from build123d import *

# Parameters (mm, degrees)
BOSS_EXTRUDE1_DEPTH = 4.7498
SKETCH2_R           = 5.715
BOSS_EXTRUDE2_DEPTH = 4.7498
SKETCH3_W           = 112.522
SKETCH3_H           = 50.8
SKETCH3_W_2         = 88.835533053
BOSS_EXTRUDE3_DEPTH = 228.6


with BuildPart() as part:
    # Sketch1 → Boss-Extrude1 (new body)
    with BuildSketch(Plane(origin=(0, 0, 0), x_dir=(1, 0, 0), z_dir=(0, 1, 0))):
        Polygon((23.686466947, -292.1), (112.522, -292.1), (112.522, -139.7), (-61.722, 292.1), (-112.522, 292.1), (-112.522, 0), align=None)
    extrude(amount=BOSS_EXTRUDE1_DEPTH)



with BuildPart() as body_2:
    # Sketch2 → Boss-Extrude2 (new body)
    with BuildSketch(Plane(origin=(-112.522, 0, 11.737401462), x_dir=(0, 0, -1), z_dir=(1, 0, 0))):
        Polygon((176.837401462, 4.7498), (231.249840519, 42.8498), (303.837401462, 42.8498), (303.837401462, 4.7498), align=None)
        with Locations(Location((291.137401462, 23.7998, 0), (0, 0, 180))):
            Circle(SKETCH2_R, mode=Mode.SUBTRACT)
        with Locations(Location((240.337401462, 23.7998, 0), (0, 0, 180))):
            Circle(SKETCH2_R, mode=Mode.SUBTRACT)
    extrude(amount=BOSS_EXTRUDE2_DEPTH)


with BuildPart() as part_1:
    add(part.part)

    add(body_2.part)  # Boss-Extrude3 merges body 2
    # Sketch3 → Boss-Extrude3 (add)
    with BuildSketch(Plane(origin=(0, 4.7498, 0), x_dir=(1, 0, 0), z_dir=(0, 1, 0))):
        with Locations((-56.261, 139.7)):
            Rectangle(SKETCH3_W, SKETCH3_H)
        with Locations((68.104233474, -266.7)):
            Rectangle(SKETCH3_W_2, SKETCH3_H)
    extrude(amount=BOSS_EXTRUDE3_DEPTH)

    # Mirror1: part across plane


with BuildPart() as part_2:
    add(part_1.part)
    add(part_1.part.mirror(Plane.ZX.offset(233.3498)))


solid = part_2.part
For this review, take the finished solid that the model builds, in its own axes (mm). A direction names the side the tool comes from. Give positions to 0.01 mm unless a question says otherwise; leave off trailing zeros. Loops run counter-clockwise (first coordinate to the right, second up) from the corner with the lowest first, then second, coordinate; pieces in that order, holes last.
Item 1: Tool access review of faces 4 (the flat face through (-71, 4.75, -229)), 5 (the flat face through (-110.18, 23.533, -191.925)), 6 (the flat face through (67, 237, 241.3)): name each direction out of +Z, -Z, +X, -X, +Y, -Y from which nothing blocks a thin tool from reaching the whole face with its end or side.
Item 2: Take a section at B-B, the plane x = -78.5. State the section outline as (y, z) points.
Item 3: Take a section at A-A, the plane z = -253. State the section outline as (x, y) points, and give its area (3 significant figures).
Item 4: Draft analysis for pull direction Y (two halves, no side actions). For faces 1 (the flat face through (-2, 0, -4)), 2 (the flat face through (-71, 461.95, -229)), 3 (the flat face through (-45.37, 2.34, 144.01)), state which applies: +Y half, -Y half, draft (parallel to the pull), parting line (faces both ways), or undercut.
Item 5: Take a section at C-C, the plane z = -150.5. State the section outline as (x, y) points.
Item 6: Take a section at D-D, the plane z = 92. State the section outline as (x, y) points, and give its area (3 significant figures).
Item 7: For line 1 along Y through (x, z) = (-108, -279); line 2 along Y through (x, z) = (-103, -238); line 3 along X through (y, z) = (295.5, -139.5), list the stretches that pass through material, from the lowest coordinate up.
Item 8: Insertion check: pin 1 (15 mm diameter, centred on y = 272, z = 276.5, fed in from -X); pin 2 (10.5 mm diameter, centred on y = 23.8, z = -228.6, fed in from -X); pin 3 (15 mm diameter, centred on y = 442.9, z = -279.4, fed in from +X); pin 4 (8 mm diameter, centred on x = -72, y = 129, fed in from +Z). Each pin has a flat end and moves straight along its axis. Give the tip position at first contact, or say it passes through.
Calculated:
1. face 4: -Z, +X
1. face 5: +X, -X
1. face 6: -Z, +X, -X
2. outline: (0, -292.1) - (4.75, -292.1) - (4.75, -165.1) - (461.95, -165.1) - (461.95, -292.1) - (466.7, -292.1) - (466.7, 72.96) - (461.95, 72.96) - (461.95, -114.3) - (4.75, -114.3) - (4.75, 72.96) - (0, 72.96) - close
3. outline: (-112.52, 0) - (-45.94, 0) - (-45.94, 4.75) - (-107.77, 4.75) - (-107.77, 42.85) - (-112.52, 42.85) - close; (-112.52, 423.85) - (-107.77, 423.85) - (-107.77, 461.95) - (-45.94, 461.95) - (-45.94, 466.7) - (-112.52, 466.7) - close
3. area: 994 mm2
4. face 1: -Y half
4. face 2: undercut
4. face 3: draft
5. outline: (-112.52, 0) - (-4.58, 0) - (-4.58, 4.75) - (0, 4.75) - (0, 461.95) - (-4.58, 461.95) - (-4.58, 466.7) - (-112.52, 466.7) - close
6. outline: (-69.62, 0) - (93.27, 0) - (93.27, 4.75) - (-69.62, 4.75) - close; (-69.62, 461.95) - (93.27, 461.95) - (93.27, 466.7) - (-69.62, 466.7) - close
6. area: 1,550 mm2
7. line 1: y = 0 to 18.1, 29.5 to 42.85, 423.85 to 437.2, 448.6 to 466.7
7. line 2: y = 0 to 4.75, 461.95 to 466.7
7. line 3: x = -112.52 to 0
8. pin 1: stops at x = 23.69
8. pin 2: passes through
8. pin 3: stops at x = -107.77
8. pin 4: stops at z = -114.3
